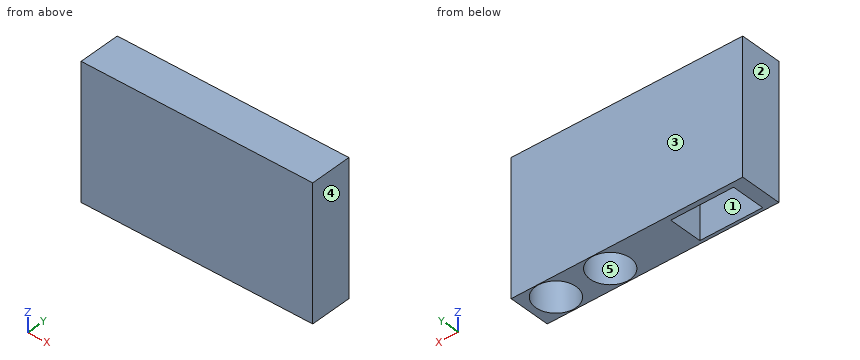
```python
from build123d import *

# Parameters (mm, degrees)
F0_W     = 140.904985
F0_H     = 81.648435
F1_DEPTH = 25.4
F2_R     = 12.273047
F2_R_2   = 12.288223
F2_W     = 38.230037
F2_H     = 20.480374
F3_DEPTH = 43.692471


with BuildPart() as f1:
    # F0 (on Front) → F1 (new body)
    with BuildSketch(Plane.XZ):
        with Locations((2.457645, -2.867254)):
            Rectangle(F0_W, F0_H)
    extrude(amount=F1_DEPTH)

    # F2 (on Top) → F3 (cut, through all)
    with BuildSketch(Plane.XY):
        with Locations((56.525838, -12.561298)):
            Circle(F2_R)
        with Locations((23.484165, -12.561298)):
            Circle(F2_R_2)
        with Locations((-40.687681, -13.243976)):
            Rectangle(F2_W, F2_H)
    extrude(amount=-F3_DEPTH, mode=Mode.SUBTRACT)


solid = f1.part
```
The model under review builds one solid part; all positions refer to its coordinate system, in mm. Face numbers are marked on the shaded views. A direction names the side the tool comes from. Coordinates: 2 decimals unless noted, no trailing zeros. Loops run counter-clockwise (first coordinate to the right, second up) from the corner with the lowest first, then second, coordinate; pieces in that order, holes last. Notation, with made-up numbers: (56.5, 27.5) -> (65.5, 27.5) arc R25 ccw to (65.5, 49.5) -> close; hole circle Ø3 at (17, -24). An arc over 180 degrees is marked (long way). Answer as CSV lines item,"result".
Item 1: Insertion check: pin 1 (12.5 mm diameter, centred on x = 18.5, y = -11.5, fed in from -Z). The pin has a flat end and moves straight along its axis. Give the tip position at first contact, or say it passes through.
Results below:
pin 1,"stops at z = 0"
Item 2: Draft analysis for pull direction Y (two halves, no side actions). For the marked faces 3, 4 and 5, state which applies: +Y half, -Y half, draft (parallel to the pull), parting line (faces both ways), or undercut.
Results below:
face 3,"+Y half"
face 4,"draft"
face 5,"undercut"
Item 3: Take a section at A-A, the plane x = -55.5. State the section outline as (y, z) points, and give its area (3 significant figures).
Results below:
outline,"(-25.4, -43.69) -> (-23.48, -43.69) -> (-23.48, 0) -> (-3, 0) -> (-3, -43.69) -> (0, -43.69) -> (0, 37.96) -> (-25.4, 37.96) -> close"
area,"1,180 mm2"
Item 4: For L1, parallel to X at y = -11.75, z = -12.5; L2, parallel to Y at x = -37, z = -35.5; L3, parallel to X at y = -18.25, z = -33, list the stretches that pass through material, from the lowest coordinate up.
Results below:
L1,"x = -67.99 to -59.8, -21.57 to 11.22, 35.75 to 44.28, 68.77 to 72.91"
L2,"y = -25.4 to -23.48, -3 to 0"
L3,"x = -67.99 to -59.8, -21.57 to 12.59, 34.38 to 45.65, 67.4 to 72.91"
Item 5: Take a section at D-D, the plane x = 16. State the section outline as (y, z) points, and give its area (3 significant figures).
Results below:
outline,"(-25.4, -43.69) -> (-22.31, -43.69) -> (-22.31, 0) -> (-2.82, 0) -> (-2.82, -43.69) -> (0, -43.69) -> (0, 37.96) -> (-25.4, 37.96) -> close"
area,"1,220 mm2"
Item 6: Take a section at C-C, the plane y = -16.5. State the section outline as (x, z) points, and give its area (3 significant figures).
Results below:
outline,"(-67.99, -43.69) -> (-59.8, -43.69) -> (-59.8, 0) -> (-21.57, 0) -> (-21.57, -43.69) -> (11.84, -43.69) -> (11.84, 0) -> (35.12, 0) -> (35.12, -43.69) -> (44.9, -43.69) -> (44.9, 0) -> (68.15, 0) -> (68.15, -43.69) -> (72.91, -43.69) -> (72.91, 37.96) -> (-67.99, 37.96) -> close"
area,"7,800 mm2"
Item 7: Take a section at B-B, the plane z = -22.5. State the section outline as (x, y) points.
Results below:
outline,"(-67.99, -25.4) -> (72.91, -25.4) -> (72.91, 0) -> (-67.99, 0) -> close; hole (-59.8, -23.48) -> (-21.57, -23.48) -> (-21.57, -3) -> (-59.8, -3) -> close; hole circle Ø24.58 at (23.48, -12.56); hole circle Ø24.55 at (56.53, -12.56)"
Item 8: Machinability: for the marked faces 1 and 2, which of the approach directions +Z, -Z, +X, -X, +Y, -Y give a long, thin tool a straight path to every point of the face, cutting with its end or side? Answer none if there is none.
Results below:
face 1,"-Z"
face 2,"+Z, -Z, -X, +Y, -Y"
